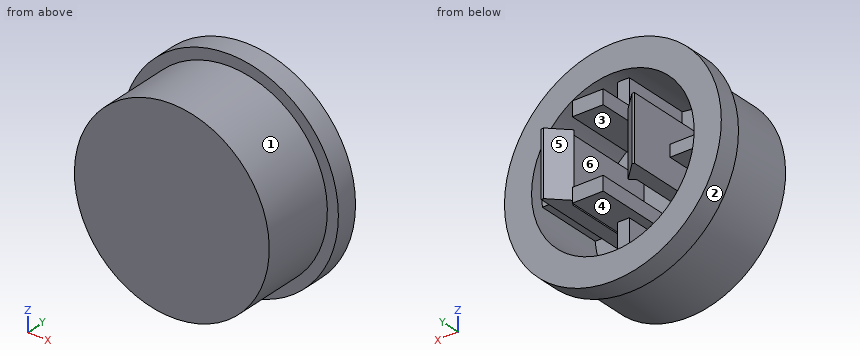
from build123d import *

# Parameters (mm, degrees)
SKETCH_1_R          = 5.75
EXTRUDE_1_DEPTH     = 0.9
SKETCH_2_R          = 5.75
SKETCH_2_R_2        = 4.8
EXTRUDE_2_DEPTH     = 3.5
SKETCH_3_R          = 6.4
SKETCH_3_R_2        = 4.8
EXTRUDE_3_DEPTH     = 1.3
SKETCH_4_W          = 0.85
SKETCH_4_H          = 3.8
SKETCH_4_W_2        = 1.824882422
SKETCH_4_H_2        = 0.85
EXTRUDE_4_DEPTH     = 6.7
EXTRUDE_5_DEPTH     = 3.8
CUT_EXTRUDE_1_REACH = 14.946
EXTRUDE_6_DEPTH     = 4


with BuildPart() as part:
    # Эскиз1 → Бобышка-Вытянуть1 (new body)
    with BuildSketch(Plane(origin=(0, 0, 0), x_dir=(1, 0, 0), z_dir=(0, 1, 0))):
        with Locations(Location((0, 0, 0), (0, 0, 270))):
            Circle(SKETCH_1_R)
    extrude(amount=EXTRUDE_1_DEPTH)

    # Эскиз2 → Бобышка-Вытянуть2 (add)
    with BuildSketch(Plane(origin=(0, 0.9, 0), x_dir=(1, 0, 0), z_dir=(0, 1, 0))):
        with Locations(Location((0, 0, 0), (0, 0, 270))):
            Circle(SKETCH_2_R)
        with Locations(Location((0, 0, 0), (0, 0, 270))):
            Circle(SKETCH_2_R_2, mode=Mode.SUBTRACT)
    extrude(amount=EXTRUDE_2_DEPTH)

    # Эскиз3 → Бобышка-Вытянуть3 (add)
    with BuildSketch(Plane(origin=(0, 4.4, 0), x_dir=(1, 0, 0), z_dir=(0, 1, 0))):
        with Locations(Location((0, 0, 0), (0, 0, 270))):
            Circle(SKETCH_3_R)
        with Locations(Location((0, 0, 0), (0, 0, 270))):
            Circle(SKETCH_3_R_2, mode=Mode.SUBTRACT)
    extrude(amount=EXTRUDE_3_DEPTH)

    # Эскиз4 → Бобышка-Вытянуть4 (add)
    with BuildSketch(Plane(origin=(0, 0.9, 0), x_dir=(1, 0, 0), z_dir=(0, 1, 0))):
        with Locations((-2.325, 0)):
            Rectangle(SKETCH_4_W, SKETCH_4_H)
        with Locations((2.325, 0)):
            Rectangle(SKETCH_4_W, SKETCH_4_H)
        with Locations((0, 2.325)):
            Rectangle(SKETCH_4_W_2, SKETCH_4_H_2)
        with Locations((0, -2.325)):
            Rectangle(SKETCH_4_W_2, SKETCH_4_H_2)
    extrude(amount=EXTRUDE_4_DEPTH)

    # Эскиз5 → Бобышка-Вытянуть5 (add)
    with BuildSketch(Plane(origin=(0, 0, -1.9), x_dir=(-1, 0, 0), z_dir=(0, 0, -1))):
        Polygon((1.9, 6.3), (1.6, 6.6), (2.6, 7.6), align=None)
        Polygon((-1.9, 6.3), (-1.6, 6.6), (-2.6, 7.6), align=None)
    extrude(amount=-EXTRUDE_5_DEPTH)

    # Эскиз6 → Вырез-Вытянуть1 (cut, up to next)
    with BuildSketch(Plane(origin=(0, 0, -1.9), x_dir=(-1, 0, 0), z_dir=(0, 0, -1)), mode=Mode.PRIVATE) as cut_extrude_1_sk1:
        Polygon((1.9, 6.9), (2.6, 7.6), (1.9, 7.6), align=None)
    cut_extrude_1_tool1 = extrude(cut_extrude_1_sk1.sketch, amount=-CUT_EXTRUDE_1_REACH, mode=Mode.PRIVATE) & part.part
    # Эскиз6 → Вырез-Вытянуть1 (cut, up to next)
    with BuildSketch(Plane(origin=(0, 0, -1.9), x_dir=(-1, 0, 0), z_dir=(0, 0, -1)), mode=Mode.PRIVATE) as cut_extrude_1_sk2:
        Polygon((-1.9, 6.9), (-2.6, 7.6), (-1.9, 7.6), align=None)
    cut_extrude_1_tool2 = extrude(cut_extrude_1_sk2.sketch, amount=-CUT_EXTRUDE_1_REACH, mode=Mode.PRIVATE) & part.part
    add(cut_extrude_1_tool1.solids().sort_by_distance((-2.133333, 7.366667, -1.9))[0], mode=Mode.SUBTRACT)
    add(cut_extrude_1_tool2.solids().sort_by_distance((2.133333, 7.366667, -1.9))[0], mode=Mode.SUBTRACT)

    # Эскиз7 → Бобышка-Вытянуть6 (add)
    with BuildSketch(Plane(origin=(0, 0.9, 0), x_dir=(1, 0, 0), z_dir=(0, 1, 0))):
        with BuildLine():
            Line((-0.35, -2.75), (0.35, -2.75))
            Line((0.35, -2.75), (0.35, -4.787222577))
            ThreePointArc((0.35, -4.787222577), (0, -4.8), (-0.35, -4.787222577))
            Line((-0.35, -4.787222577), (-0.35, -2.75))
        make_face()
        with BuildLine():
            Line((4.787222577, -0.35), (2.75, -0.35))
            Line((2.75, -0.35), (2.75, 0.35))
            Line((2.75, 0.35), (4.787222577, 0.35))
            ThreePointArc((4.787222577, 0.35), (4.8, 0), (4.787222577, -0.35))
        make_face()
        with BuildLine():
            Line((0.35, 2.75), (0.35, 4.787222577))
            ThreePointArc((0.35, 4.787222577), (0, 4.8), (-0.35, 4.787222577))
            Line((-0.35, 4.787222577), (-0.35, 2.75))
            Line((-0.35, 2.75), (0.35, 2.75))
        make_face()
        with BuildLine():
            Line((-2.75, -0.35), (-4.787222577, -0.35))
            ThreePointArc((-4.787222577, -0.35), (-4.8, 0), (-4.787222577, 0.35))
            Line((-4.787222577, 0.35), (-2.75, 0.35))
            Line((-2.75, 0.35), (-2.75, -0.35))
        make_face()
    extrude(amount=EXTRUDE_6_DEPTH)


solid = part.part
Source: CAD feature listing. Evaluate the final solid. Frame: model axes, mm. Face numbers are marked on the shaded views. A direction names the side the tool comes from. Give positions to 0.01 mm unless a question says otherwise; leave off trailing zeros. Order: outer loops, then holes, each group sorted by start corner. A loop starts at its lowest first (then second) coordinate and runs counter-clockwise, first axis right, second up. Notation, with made-up numbers: (36.25, -35.75) -> (94.25, -35.75) arc R22 ccw to (94.25, 0.25) -> close; hole circle Ø6 at (59.25, -27). An arc over 180 degrees is marked (long way). Use a Markdown table: item, result.
1) Section query C-C, the plane z = 0. Return the cut outline in (x, y), then the cut area to 3 significant figures.
Answer list:
| item | result |
|---|---|
| outline | (-6.4, 4.4) -> (-5.75, 4.4) -> (-5.75, 0) -> (5.75, 0) -> (5.75, 4.4) -> (6.4, 4.4) -> (6.4, 5.7) -> (4.8, 5.7) -> (4.8, 4.9) -> (2.75, 4.9) -> (2.75, 7.6) -> (2.6, 7.6) -> (1.6, 6.6) -> (1.9, 6.3) -> (1.9, 0.9) -> (-1.9, 0.9) -> (-1.9, 6.3) -> (-1.6, 6.6) -> (-2.6, 7.6) -> (-2.75, 7.6) -> (-2.75, 4.9) -> (-4.8, 4.9) -> (-4.8, 5.7) -> (-6.4, 5.7) -> close |
| area | 48.6 mm² |
2) Ray query, line 1 along Z through (x, y) = (-0.5, 5.75); line 2 along X through (y, z) = (1, -0.75). Return the intervals inside material, ascending. Write a range as [from, to].
Answer list:
| item | result |
|---|---|
| line 1 | [-2.75, -1.9], [1.9, 2.75] |
| line 2 | [-5.7, -4.74], [-2.75, -1.9], [1.9, 2.75], [4.74, 5.7] |
3) Contact query for flat-ended pins moving along their axis: P1, Ø2, axis at x = 3.5, z = 4, coming from the +Y side; P2, Ø1.5, axis at x = -4, y = 4, coming from the +Z side; P3, Ø1.6, axis at x = -4, y = 2, coming from the -Z side. Output: stop coordinate, or through.
Answer list:
| item | result |
|---|---|
| P1 | y = 5.7 |
| P2 | z = 5.44 |
| P3 | z = -4.78 |
4) Reachability of the marked faces 1, 2 and 3 from +Z, -Z, +X, -X, +Y, -Y: full face, straight path, thin tool, end or side. Return the list, or none.
Answer list:
| item | result |
|---|---|
| face 1 | -Y |
| face 2 | +Y, -Y |
| face 3 | +Y |
5) Mould query, pull axis Y, two halves, no side actions, for the marked faces 4, 5 and 6. Classes: +Y half, -Y half, draft (parallel to the pull), parting line (faces both ways), or undercut.
Answer list:
| item | result |
|---|---|
| face 4 | draft |
| face 5 | +Y half |
| face 6 | undercut |
6) Section query D-D, the plane x = 0. Return the cut outline in (y, z).
Answer list:
| item | result |
|---|---|
| outline | (0, -5.75) -> (4.4, -5.75) -> (4.4, -6.4) -> (5.7, -6.4) -> (5.7, -4.8) -> (4.9, -4.8) -> (4.9, -2.75) -> (7.6, -2.75) -> (7.6, -1.9) -> (0.9, -1.9) -> (0.9, 1.9) -> (7.6, 1.9) -> (7.6, 2.75) -> (4.9, 2.75) -> (4.9, 4.8) -> (5.7, 4.8) -> (5.7, 6.4) -> (4.4, 6.4) -> (4.4, 5.75) -> (0, 5.75) -> close |
7) Section query A-A, the plane y = 5.5. Return the cut outline in (x, z), then the cut area to 3 significant figures.
Answer list:
| item | result |
|---|---|
| outline | circle Ø12.8 at (0, 0); (-2.75, -1.9) -> (-1.9, -1.9) -> (-1.9, 1.9) -> (-2.75, 1.9) -> close; (-0.91, -2.75) -> (0.91, -2.75) -> (0.91, -1.9) -> (-0.91, -1.9) -> close; (-0.91, 1.9) -> (0.91, 1.9) -> (0.91, 2.75) -> (-0.91, 2.75) -> close; (1.9, -1.9) -> (2.75, -1.9) -> (2.75, 1.9) -> (1.9, 1.9) -> close; hole circle Ø9.6 at (0, 0) |
| area | 65.9 mm² |
